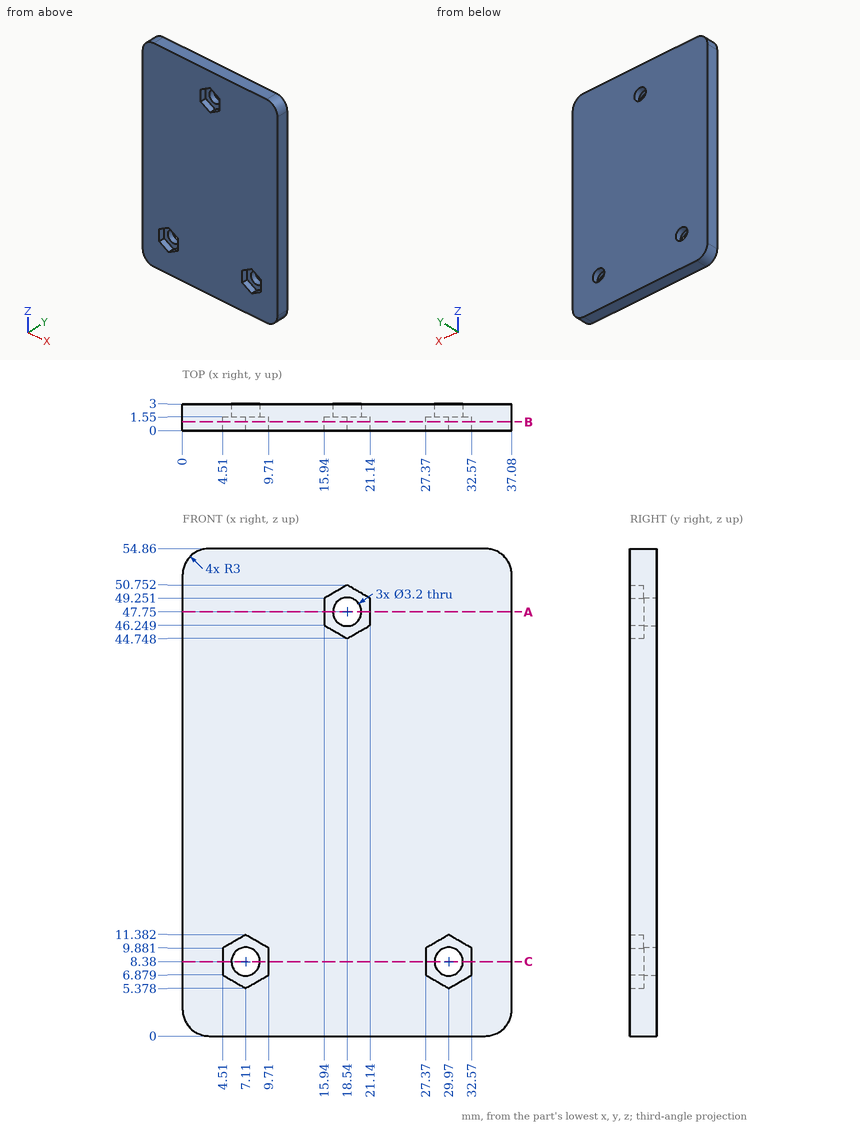
Print and shaded views of the part. All mm, measured from the part's lowest x, y and z. Round coordinates to 2 decimals unless told otherwise and drop trailing zeros. Write each loop counter-clockwise with the first axis right and the second up, starting at its lowest first coordinate (ties: lowest second). Pieces come first, ordered by that corner, then holes.
Item 1: Probe L1, parallel to X at y = 2.7, z = 8.38; L2, parallel to X at y = 2.15, z = 47.75; L3, parallel to Z at x = 18, y = 2. List the from-to ranges inside material, lowest first.
Results:
L1: x = 0 to 5.51, 8.71 to 28.37, 31.57 to 37.08
L2: x = 0 to 16.94, 20.14 to 37.08
L3: z = 0 to 46.24, 49.26 to 54.86
Item 2: Cut at C-C, the plane z = 8.38. Give the cut face in (x, y).
Results:
outline: (0, 0) - (4.51, 0) - (4.51, 1.55) - (5.51, 1.55) - (5.51, 3) - (0, 3) - close; (8.71, 1.55) - (9.71, 1.55) - (9.71, 0) - (27.37, 0) - (27.37, 1.55) - (28.37, 1.55) - (28.37, 3) - (8.71, 3) - close; (31.57, 1.55) - (32.57, 1.55) - (32.57, 0) - (37.08, 0) - (37.08, 3) - (31.57, 3) - close
Item 3: Drop flat-ended pins along their axis: pin 1 Ø2.5 at (x, z) = (30, 9) entering from -Y; pin 2 Ø2.5 at (x, z) = (18.54, 47.75) entering from +Y. Give the stop position or say it passes through.
Results:
pin 1: stops at y = 1.55
pin 2: passes through
Item 4: Cut at A-A, the plane z = 47.75. Give the cut face in (x, y).
Results:
outline: (0, 0) - (15.94, 0) - (15.94, 1.55) - (16.94, 1.55) - (16.94, 3) - (0, 3) - close; (20.14, 1.55) - (21.14, 1.55) - (21.14, 0) - (37.08, 0) - (37.08, 3) - (20.14, 3) - close
Item 5: Cut at B-B, the plane y = 1. Give the cut face in (x, z).
Results:
outline: (0, 3) arc R3 ccw to (3, 0) - (34.08, 0) arc R3 ccw to (37.08, 3) - (37.08, 51.86) arc R3 ccw to (34.08, 54.86) - (3, 54.86) arc R3 ccw to (0, 51.86) - close; hole (4.51, 6.88) - (7.11, 5.38) - (9.71, 6.88) - (9.71, 9.88) - (7.11, 11.38) - (4.51, 9.88) - close; hole (15.94, 46.25) - (18.54, 44.75) - (21.14, 46.25) - (21.14, 49.25) - (18.54, 50.75) - (15.94, 49.25) - close; hole (27.37, 6.88) - (29.97, 5.38) - (32.57, 6.88) - (32.57, 9.88) - (29.97, 11.38) - (27.37, 9.88) - close
